```python
from build123d import *

# Parameters (mm, degrees)
F1_R      = 2.75
F1_R_2    = 2
F2_DEPTH  = 5.4
F4_R      = 7.7
F4_R_2    = 2
F5_DEPTH  = 1
F8_DEPTH  = 213
F11_DEPTH = 3.5
F12_SIZE  = 1.65
F13_SIZE  = 0.2


with BuildPart() as f2:
    # F1 (on offset) → F2 (new body)
    with BuildSketch(Plane.XY.offset(13)):
        Circle(F1_R)
        Circle(F1_R_2, mode=Mode.SUBTRACT)
    extrude(amount=-F2_DEPTH)

    # F4 (on offset) → F5 (join)
    with BuildSketch(Plane.XY.offset(13)):
        Circle(F4_R)
        Circle(F4_R_2, mode=Mode.SUBTRACT)
    extrude(amount=-F5_DEPTH)

    # F7 (on offset) → F8 (cut)
    with BuildSketch(Plane.XY.offset(13)):
        with BuildLine():
            Line((-0.5, 6), (-0.5, 7.683749))
            ThreePointArc((-0.5, 7.683749), (-2.792892, 7.175636), (-4.825971, 6))
            Line((-4.825971, 6), (-0.5, 6))
        make_face()
        with BuildLine():
            Line((-6, -0.5), (-7.683749, -0.5))
            ThreePointArc((-7.683749, -0.5), (-7.175636, -2.792892), (-6, -4.825971))
            Line((-6, -4.825971), (-6, -0.5))
        make_face()
        with BuildLine():
            Line((0.5, -6), (0.5, -7.683749))
            ThreePointArc((0.5, -7.683749), (2.792892, -7.175636), (4.825971, -6))
            Line((4.825971, -6), (0.5, -6))
        make_face()
        with BuildLine():
            ThreePointArc((7.683749, 0.5), (7.175636, 2.792892), (6, 4.825971))
            Line((6, 4.825971), (6, 0.5))
            Line((6, 0.5), (7.683749, 0.5))
        make_face()
    extrude(amount=-F8_DEPTH, mode=Mode.SUBTRACT)

    # F10 (on offset) → F11 (join)
    with BuildSketch(Plane.XY.offset(12)):
        with BuildLine():
            Line((-6, 0.5), (-7.683749, 0.5))
            ThreePointArc((-7.683749, 0.5), (-7.7, 0), (-7.683749, -0.5))
            Line((-7.683749, -0.5), (-6, -0.5))
            Line((-6, -0.5), (-6, 0.5))
        make_face()
        with BuildLine():
            ThreePointArc((0.5, 7.683749), (0, 7.7), (-0.5, 7.683749))
            Line((-0.5, 7.683749), (-0.5, 6))
            Line((-0.5, 6), (0.5, 6))
            Line((0.5, 6), (0.5, 7.683749))
        make_face()
        with BuildLine():
            Line((7.683749, 0.5), (6, 0.5))
            Line((6, 0.5), (6, -0.5))
            Line((6, -0.5), (7.683749, -0.5))
            ThreePointArc((7.683749, -0.5), (7.7, 0), (7.683749, 0.5))
        make_face()
        with BuildLine():
            ThreePointArc((-0.5, -7.683749), (0, -7.7), (0.5, -7.683749))
            Line((0.5, -7.683749), (0.5, -6))
            Line((0.5, -6), (-0.5, -6))
            Line((-0.5, -6), (-0.5, -7.683749))
        make_face()
    extrude(amount=-F11_DEPTH)

    # F12
    f12_edges = [f2.edges().sort_by_distance(p)[0] for p in [
        (-6, 0, 8.5),
        (0, 6, 8.5),
        (6, 0, 8.5),
        (0, -6, 8.5),
    ]]
    chamfer(f12_edges, length=F12_SIZE)

    # F13
    f13_edges = [f2.edges().sort_by_distance(p)[0] for p in [
        (-2, 0, 13),
    ]]
    chamfer(f13_edges, length=F13_SIZE)


solid = f2.part
```
Part model, mm, in its own coordinate system. A direction names the side the tool comes from. Round coordinates to 2 decimals unless told otherwise and drop trailing zeros. Order: outer loops, then holes, each group sorted by start corner. A loop starts at its lowest first (then second) coordinate and runs counter-clockwise, first axis right, second up. Notation, with made-up numbers: M 66.25,-2 L 101.25,-2 A22 ccw 101.25,8 Z; hole C -31,-0.75 d7. An arc over 180 degrees is marked long. Put each result on its own line as item: value. Start each with the question number.
1. Drill centre lines: probe 1 along Y at (x, z) = (0, 11.4); probe 2 along Y at (x, z) = (0, 8.8); probe 3 along Z at (x, y) = (-3.5, -5.5). Where is each one in solid material? Low to high. Write a range as [from, to].
2. Tool access for faces 4 (the face through (7, -0.5, 11)), 5 (the face through (-6, 0, 11)), 6 (the face through (-7, 0.5, 11)), 7 (the face through (-7, -0.5, 11)): list every direction of +Z, -Z, +X, -X, +Y, -Y with a clear straight run to the whole face (end or side of a thin tool).
3. Slice it at D-D on z = 10.5. List the corners of the cut face in (x, y).
4. Drop flat-ended pins along their axis: pin 1 (0.5 mm diameter, centred on x = -7, z = 10.5, fed in from +Y); pin 2 (0.8 mm diameter, centred on x = 3, z = 12.5, fed in from -Y); pin 3 (0.5 mm diameter, centred on x = -3, z = 12.5, fed in from +Y). Give the stop position or say it passes through.
5. Two-plate mould, pull along X, no slides. Class faces 1 (the face through (-6.84, -0.01, 9.31)), 2 (the face through (-2.7, 6, 12.5)), 3 (the face through (-7.028, 3.146, 12.507)): +X half, -X half, draft (parallel to the pull), parting line (faces both ways), or undercut.
6. Slice it at A-A on z = 9.45. List the corners of the cut face in (x, y).
7. Slice it at B-B on x = 0. List the corners of the cut face in (y, z).
Findings:
1. probe 1: [-7.7, -6], [-2.75, -2], [2, 2.75], [6, 7.7]
1. probe 2: [-7.7, -7.35], [-2.75, -2], [2, 2.75], [7.35, 7.7]
1. probe 3: [12, 13]
2. face 4: -Z, +X, -Y
2. face 5: -Z, +Y, -Y
2. face 6: -Z, -X, +Y
2. face 7: +Z, -Z, -X, -Y
3. outline: M -7.68,-0.5 L -6,-0.5 L -6,0.5 L -7.68,0.5 A7.7 ccw Z; C 0,0 d5.5; M -0.5,-7.68 A7.7 ccw 0.5,-7.68 L 0.5,-6 L -0.5,-6 Z; M -0.5,6 L 0.5,6 L 0.5,7.68 A7.7 ccw -0.5,7.68 Z; M 6,-0.5 L 7.68,-0.5 A7.7 ccw 7.68,0.5 L 6,0.5 Z; hole C 0,0 d4
4. pin 1: y = 0.5
4. pin 2: y = -6
4. pin 3: y = 6
5. face 1: undercut
5. face 2: draft
5. face 3: -X half
6. outline: M -7.68,-0.5 L -6.7,-0.5 L -6.7,0.5 L -7.68,0.5 A7.7 ccw Z; C 0,0 d5.5; M -0.5,-7.68 A7.7 ccw 0.5,-7.68 L 0.5,-6.7 L -0.5,-6.7 Z; M -0.5,6.7 L 0.5,6.7 L 0.5,7.68 A7.7 ccw -0.5,7.68 Z; M 6.7,-0.5 L 7.68,-0.5 A7.7 ccw 7.68,0.5 L 6.7,0.5 Z; hole C 0,0 d4
7. outline: M -7.7,8.5 L -7.65,8.5 L -6,10.15 L -6,12 L -2.75,12 L -2.75,7.6 L -2,7.6 L -2,12.8 L -2.2,13 L -7.7,13 Z; M 2,7.6 L 2.75,7.6 L 2.75,12 L 6,12 L 6,10.15 L 7.65,8.5 L 7.7,8.5 L 7.7,13 L 2.2,13 L 2,12.8 Z
